from build123d import *

# Parameters (mm, degrees)
F0_R     = 1.5
F1_DEPTH = 7


with BuildPart() as f1:
    # F0 (on Front) → F1 (new body)
    with BuildSketch(Plane.XZ):
        with BuildLine():
            Line((-39, 0), (0, 0))
            Line((0, 0), (24, 0))
            ThreePointArc((24, 0), (24.707107, 0.292893), (25, 1))
            Line((25, 1), (25, 2.112826))
            ThreePointArc((25, 2.112826), (24.748046, 2.776473), (24.119145, 3.105703))
            Line((24.119145, 3.105703), (1.483992, 5.821921))
            ThreePointArc((1.483992, 5.821921), (-0.002664, 5.955441), (-1.494639, 6))
            Line((-1.494639, 6), (-4.226051, 6))
            ThreePointArc((-4.226051, 6), (-4.916289, 5.877118), (-5.521709, 5.523571))
            ThreePointArc((-5.521709, 5.523571), (-12, 3.141428), (-18.478291, 5.523571))
            ThreePointArc((-18.478291, 5.523571), (-19.083711, 5.877118), (-19.773949, 6))
            Line((-19.773949, 6), (-24.02225, 6))
            ThreePointArc((-24.02225, 6), (-24.8413, 5.824598), (-25.516687, 5.329156))
            ThreePointArc((-25.516687, 5.329156), (-30, 3.316625), (-34.483313, 5.329156))
            ThreePointArc((-34.483313, 5.329156), (-35.1587, 5.824598), (-35.97775, 6))
            Line((-35.97775, 6), (-39, 6))
            ThreePointArc((-39, 6), (-39.707107, 5.707107), (-40, 5))
            Line((-40, 5), (-40, 1))
            ThreePointArc((-40, 1), (-39.707107, 0.292893), (-39, 0))
        make_face()
        with Locations((-37, 3)):
            Circle(F0_R, mode=Mode.SUBTRACT)
    extrude(amount=F1_DEPTH)


solid = f1.part
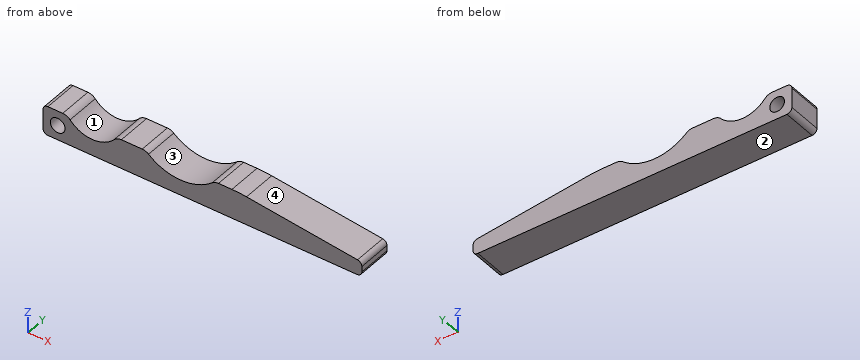
Design review of the part built by this model. Coordinates are the model's own, in mm. Face numbers are marked on the shaded views. Give positions to 0.01 mm unless a question says otherwise; leave off trailing zeros. Loops run counter-clockwise (first coordinate to the right, second up) from the corner with the lowest first, then second, coordinate; pieces in that order, holes last. Notation, with made-up numbers: M 75,-33 L 98,-33 A17 ccw 98,-22 Z; hole C 10.5,-28.5 d6. An arc over 180 degrees is marked long. Write item = value, one per line.
Q1. Draft analysis for pull direction X (two halves, no side actions). For the marked faces 1, 2, 3 and 4, state which applies: +X half, -X half, draft (parallel to the pull), parting line (faces both ways), or undercut.
Output values:
face_1 = undercut
face_2 = draft
face_3 = undercut
face_4 = +X half
Q2. We need section D-D (x = -29.5). Give the boundary of the cut face in (y, z), plus the area to 3 significant figures.
Output values:
outline = M -7,0 L 0,0 L 0,3.34 L -7,3.34 Z
area = 23.4 mm^2
Q3. We need section A-A (x = -37). Give the boundary of the cut face in (y, z), plus the area to 3 significant figures.
Output values:
outline = M -7,0 L 0,0 L 0,1.5 L -7,1.5 Z; M -7,4.5 L 0,4.5 L 0,6 L -7,6 Z
area = 21.0 mm^2
Q4. We need section C-C (x = 19). Give the boundary of the cut face in (y, z).
Output values:
outline = M -7,0 L 0,0 L 0,3.72 L -7,3.72 Z
Q5. We need section B-B (y = -3.75). Give the boundary of the cut face in (x, z).
Output values:
outline = M -40,1 A1 ccw -39,0 L 24,0 A1 ccw 25,1 L 25,2.11 A1 ccw 24.12,3.11 L 1.48,5.82 A25 ccw -1.49,6 L -4.23,6 A2 ccw -5.52,5.52 A10 cw -18.48,5.52 A2 ccw -19.77,6 L -24.02,6 A2 ccw -25.52,5.33 A6 cw -34.48,5.33 A2 ccw -35.98,6 L -39,6 A1 ccw -40,5 Z; hole C -37,3 d3
Q6. To check wall thickness, follow line 1 (Z direction, x = -37, y = -1.5); line 2 (Z direction, x = -12.5, y = -2.5); line 3 (Z direction, x = 12, y = -1). State the ranges of each line that lie inside material, in increasing order. Write a range as [from, to].
Output values:
line_1 = [0, 1.5], [4.5, 6]
line_2 = [0, 3.15]
line_3 = [0, 4.56]
